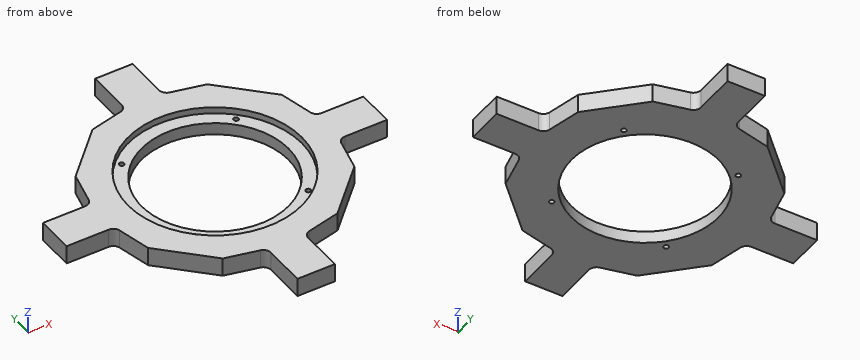
from build123d import *

# Parameters (mm, degrees)
BOSS_EXTRUDE1_DEPTH = 19.05
SKETCH2_R           = 74.93
CUT_EXTRUDE1_DEPTH  = 232.935451585
SKETCH3_R           = 88.546370902
CUT_EXTRUDE2_DEPTH  = 6.604
SKETCH4_R           = 2.5
CUT_EXTRUDE3_DEPTH  = 232.486617579


with BuildPart() as part:
    # Sketch1 → Boss-Extrude1 (new body)
    with BuildSketch(Plane.XY):
        with BuildLine():
            Line((-19.05, 120.51752167), (-19.05, 163.449))
            Line((-19.05, 163.449), (19.05, 163.449))
            Line((19.05, 163.449), (19.05, 120.51752167))
            ThreePointArc((19.05, 120.51752167), (20.700629733, 115.781382038), (24.937406462, 113.097109308))
            Line((24.937406462, 113.097109308), (58.551269909, 105.248601739))
            Line((58.551269909, 105.248601739), (105.248601739, 58.551269909))
            Line((105.248601739, 58.551269909), (113.097109308, 24.937406462))
            ThreePointArc((113.097109308, 24.937406462), (115.781382038, 20.700629733), (120.51752167, 19.05))
            Line((120.51752167, 19.05), (163.449, 19.05))
            Line((163.449, 19.05), (163.449, -19.05))
            Line((163.449, -19.05), (120.51752167, -19.05))
            ThreePointArc((120.51752167, -19.05), (115.781382038, -20.700629733), (113.097109308, -24.937406462))
            Line((113.097109308, -24.937406462), (105.248601739, -58.551269909))
            Line((105.248601739, -58.551269909), (58.551269909, -105.248601739))
            Line((58.551269909, -105.248601739), (24.937406462, -113.097109308))
            ThreePointArc((24.937406462, -113.097109308), (20.700629733, -115.781382038), (19.05, -120.51752167))
            Line((19.05, -120.51752167), (19.05, -163.449))
            Line((19.05, -163.449), (-19.05, -163.449))
            Line((-19.05, -163.449), (-19.05, -120.51752167))
            ThreePointArc((-19.05, -120.51752167), (-20.700629733, -115.781382038), (-24.937406462, -113.097109308))
            Line((-24.937406462, -113.097109308), (-58.551269909, -105.248601739))
            Line((-58.551269909, -105.248601739), (-105.248601739, -58.551269909))
            Line((-105.248601739, -58.551269909), (-113.097109308, -24.937406462))
            ThreePointArc((-113.097109308, -24.937406462), (-115.781382038, -20.700629733), (-120.51752167, -19.05))
            Line((-120.51752167, -19.05), (-163.449, -19.05))
            Line((-163.449, -19.05), (-163.449, 19.05))
            Line((-163.449, 19.05), (-120.51752167, 19.05))
            ThreePointArc((-120.51752167, 19.05), (-115.781382038, 20.700629733), (-113.097109308, 24.937406462))
            Line((-113.097109308, 24.937406462), (-105.248601739, 58.551269909))
            Line((-105.248601739, 58.551269909), (-58.551269909, 105.248601739))
            Line((-58.551269909, 105.248601739), (-24.937406462, 113.097109308))
            ThreePointArc((-24.937406462, 113.097109308), (-20.700629733, 115.781382038), (-19.05, 120.51752167))
        make_face()
    extrude(amount=BOSS_EXTRUDE1_DEPTH)

    # Sketch2 → Cut-Extrude1 (cut, through all)
    with BuildSketch(Plane.XY.offset(19.05)):
        Circle(SKETCH2_R)
    extrude(amount=-CUT_EXTRUDE1_DEPTH, mode=Mode.SUBTRACT)

    # Sketch3 → Cut-Extrude2 (cut)
    with BuildSketch(Plane.XY.offset(19.05)):
        Circle(SKETCH3_R)
    extrude(amount=-CUT_EXTRUDE2_DEPTH, mode=Mode.SUBTRACT)

    # Sketch4 → Cut-Extrude3 (cut, through all)
    with BuildSketch(Plane.XY.offset(12.446)):
        with Locations((-58.336309448, 58.336309448)):
            Circle(SKETCH4_R)
        with Locations((58.336309448, 58.336309448)):
            Circle(SKETCH4_R)
        with Locations((58.336309448, -58.336309448)):
            Circle(SKETCH4_R)
        with Locations((-58.336309448, -58.336309448)):
            Circle(SKETCH4_R)
    extrude(amount=-CUT_EXTRUDE3_DEPTH, mode=Mode.SUBTRACT)


solid = part.part
The listing builds one solid part. Answer for the finished solid, in the listing's coordinates (mm). Round coordinates to 2 decimals unless told otherwise and drop trailing zeros. Order: outer loops, then holes, each group sorted by start corner. A loop starts at its lowest first (then second) coordinate and runs counter-clockwise, first axis right, second up. Notation, with made-up numbers: M 51,46 L 77,46 A14 ccw 77,60 Z; hole C 44,-10 d5. An arc over 180 degrees is marked long. Answer in a Markdown table with one row per item. Add a question column.
1) Consider line 1 along Y through (x, z) = (0, 10); line 2 along X through (y, z) = (-3, 13.25); line 3 along X through (y, z) = (-135, 9.5). Determine where each line is inside the solid, lowest interval first. Write a range as from..to.
2) The part is cut by section A-A on y = 0. Determine the outline of the cut face in (x, z), plus the area to 3 significant figures.
3) Flat-ended cylindrical pins translate along their axes: pin 1 Ø8 at (y, z) = (81, 8.5) entering from +X; pin 2 Ø5.5 at (y, z) = (-139.5, 7) entering from -X; pin 3 Ø3 at (x, y) = (-58.34, 58.34) entering from +Z; pin 4 Ø10 at (x, z) = (77.5, 12) entering from +Y. Find the tip coordinate at first contact, or state that the pin passes through.
4) The part is cut by section D-D on x = -109. Determine the outline of the cut face in (y, z), plus the area to 3 significant figures.
Findings below:
| question | item | result |
|---|---|---|
| 1 | line 1 | y = -163.45..-74.93, 74.93..163.45 |
| 1 | line 2 | x = -163.45..-88.5, 88.5..163.45 |
| 1 | line 3 | x = -19.05..19.05 |
| 2 | outline | M -163.45,0 L -74.93,0 L -74.93,12.45 L -88.55,12.45 L -88.55,19.05 L -163.45,19.05 Z; M 74.93,0 L 163.45,0 L 163.45,19.05 L 88.55,19.05 L 88.55,12.45 L 74.93,12.45 Z |
| 2 | area | 3,190 mm² |
| 3 | pin 1 | stops at x = 86.8 |
| 3 | pin 2 | stops at x = -19.05 |
| 3 | pin 3 | passes through |
| 3 | pin 4 | stops at y = 91.3 |
| 4 | outline | M -42.48,0 L 42.48,0 L 42.48,19.05 L -42.48,19.05 Z |
| 4 | area | 1,620 mm² |
